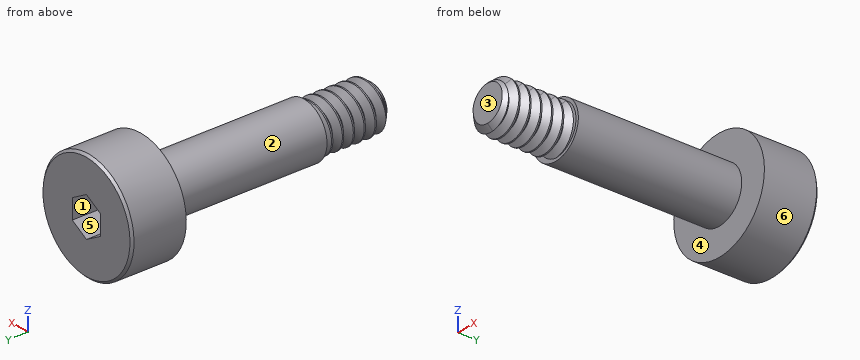
```python
from build123d import *

# Parameters (mm, degrees)
SKETCH1_R          = 3.175
EXTRUDE1_DEPTH     = 3.175
CUT_EXTRUDE1_DEPTH = 1.5875
SKETCH4_R          = 1.5875
EXTRUDE2_DEPTH     = 9.525
SKETCH5_R          = 1.4224
EXTRUDE3_DEPTH     = 3.96875
CHAMFER1_SIZE      = 0.396875
CUT_SWEEP1_PITCH   = 0.635
CUT_SWEEP1_TO      = 3.96875


with BuildPart() as part:
    # Sketch1 → Extrude1 (new body)
    with BuildSketch(Plane(origin=(0, 0, 0), x_dir=(1, 0, 0), z_dir=(0, 1, 0))):
        with Locations(Location((0, 0, 0), (0, 0, 270))):
            Circle(SKETCH1_R)
    extrude(amount=EXTRUDE1_DEPTH)

    # Sketch2 → Cut-Extrude1 (cut)
    with BuildSketch(Plane(origin=(0, 3.175, 0), x_dir=(-1, 0, 0), z_dir=(0, 1, 0))):
        Polygon((0, -1.14567944), (0.9921875, -0.57283972), (0.9921875, 0.57283972), (0, 1.14567944), (-0.9921875, 0.57283972), (-0.9921875, -0.57283972), align=None)
    extrude(amount=-CUT_EXTRUDE1_DEPTH, mode=Mode.SUBTRACT)

    # Sketch4 → Extrude2 (add)
    with BuildSketch(Plane.XZ):
        with Locations(Location((0, 0, 0), (0, 0, 90))):
            Circle(SKETCH4_R)
    extrude(amount=EXTRUDE2_DEPTH)

    # Sketch5 → Extrude3 (add)
    with BuildSketch(Plane.XZ.offset(9.525)):
        with Locations(Location((0, 0, 0), (0, 0, 270))):
            Circle(SKETCH5_R)
    extrude(amount=EXTRUDE3_DEPTH)

    # Chamfer1
    chamfer1_edges = [part.edges().sort_by_distance(p)[0] for p in [
        (0, -13.49375, 1.4224),
    ]]
    chamfer(chamfer1_edges, length=CHAMFER1_SIZE)

    # Cut-Sweep1: arcs per turn and ends read off the stored shape
    # Cut-Sweep1: the profile of Sketch13 profile screwed along a right-hand helix through 7 turns, 6 arcs to a turn; built about Z, then put on its axis
    cut_sweep1_z = Axis((0, 0, 0), (0, 0, 1))
    cut_sweep1_corners = [(1.4227, 0, -0.079201795), (1.4227, 0, -0.635173205), (1.009955401, 0, -0.396875), (1.009955401, 0, -0.3175)]
    with BuildLine(mode=Mode.PRIVATE) as cut_sweep1_profile:
        Line(cut_sweep1_corners[0], cut_sweep1_corners[1])
        Line(cut_sweep1_corners[1], cut_sweep1_corners[2])
        Line(cut_sweep1_corners[2], cut_sweep1_corners[3])
        Line(cut_sweep1_corners[3], cut_sweep1_corners[0])
    cut_sweep1_cap = Face(cut_sweep1_profile.wire())
    cut_sweep1_turn_angles = [0, 30, 60, 90, 120, 150, 180, 210, 240, 270, 300, 330, 360]
    cut_sweep1_turn_weights = [1, 0.8660254037844387, 1, 0.8660254037844387, 1, 0.8660254037844387, 1, 0.8660254037844387, 1, 0.8660254037844387, 1, 0.8660254037844387, 1]
    cut_sweep1_turn_rails = [Edge.make_bspline([Vector(p[0], p[1], 0).rotate(cut_sweep1_z, cut_sweep1_turn_angles[k]) / cut_sweep1_turn_weights[k] + Vector(0, 0, p[2] + CUT_SWEEP1_PITCH * cut_sweep1_turn_angles[k] / 360) for k in range(13)], [0, 0, 0, 1, 1, 2, 2, 3, 3, 4, 4, 5, 5, 6, 6, 6], 2, cut_sweep1_turn_weights) for p in cut_sweep1_corners]
    cut_sweep1_turn_sides = [Face.make_surface_from_curves(cut_sweep1_turn_rails[p[0]], cut_sweep1_turn_rails[p[1]]) for p in [(0, 1), (1, 2), (2, 3), (3, 0)]]
    cut_sweep1 = Plane(origin=(0, -13.49375, 0), x_dir=(0.7071067811865438, 0, 0.7071067811865512), z_dir=(0, 1, 0)) * split(Solid(Shell([*[p.moved(Location((0, 0, CUT_SWEEP1_PITCH * i))) for i in range(7) for p in cut_sweep1_turn_sides], cut_sweep1_cap, cut_sweep1_cap.rotate(cut_sweep1_z, 2520).moved(Location((0, 0, CUT_SWEEP1_PITCH * 2520 / 360)))])), bisect_by=Plane.XY.offset(CUT_SWEEP1_TO), keep=Keep.BOTTOM, mode=Mode.PRIVATE)
    add(cut_sweep1, mode=Mode.SUBTRACT)

    # Sketch11 → Cut-Revolve7 (revolve, cut)
    with BuildSketch(Plane.XY, mode=Mode.PRIVATE) as cut_revolve7_sk:
        Polygon((3.175, 3.045510577), (3.045510577, 3.175), (3.175, 3.175), align=None)
    revolve(cut_revolve7_sk.sketch.rotate(Axis((0, 14.544175091, 0), (0, -1, 0)), 90), axis=Axis((0, 14.544175091, 0), (0, -1, 0)), mode=Mode.SUBTRACT)


solid = part.part
```
Geometry check sheet. Reference: the model listing, model coordinates, mm. Face numbers are marked on the shaded views. A direction names the side the tool comes from. Coordinates: 2 decimals unless noted, no trailing zeros. Write each loop counter-clockwise with the first axis right and the second up, starting at its lowest first coordinate (ties: lowest second). Pieces come first, ordered by that corner, then holes. Notation, with made-up numbers: M 81.25,10.5 L 123.25,10.5 A23 ccw 123.25,37.5 Z; hole C 41,77 d10. An arc over 180 degrees is marked long. Use one line per item in the form item = value. Start each with the question number.
1) Thickness scan on probe 1 along Y at (x, z) = (0.75, 1.25) (3 decimals); probe 2 along Y at (x, z) = (2, -1.75) (3 decimals); probe 3 along Z at (x, y) = (-0.25, 2). Record the ranges inside material, lowest first. Write a range as from..to.
2) Release check for a two-part mould opening along X. For the marked faces 1, 2 and 3 record: pulls with the +X half, pulls with the -X half, needs draft (parallel to the pull), parting line crosses it, or undercut.
3) Section check B-B on y = 1. Enter the section's corners in (x, z) (3 decimals).
4) Set-up check for the marked faces 4, 5 and 6: record each of +Z, -Z, +X, -X, +Y, -Y from which the full face is reachable in a straight line by a thin tool's end or side.
5) Go/stop test with a flat-tipped pin: pin 1 Ø3 at (x, y) = (0, -7) entering from -Z. Record where the tip stops, or that it passes through.
6) Section check A-A on y = -7.25. Enter the section's corners in (x, z) (1 decimal), and give its area (3 significant figures).
Responses:
q1.probe_1 = -9.525..3.175
q1.probe_2 = 0..3.175
q1.probe_3 = -3.17..-1, 1..3.17
q2.face_1 = undercut
q2.face_2 = parting line crosses it
q2.face_3 = needs draft
q3.outline = C 0,0 d6.35
q4.face_4 = -Y
q4.face_5 = +Y
q4.face_6 = +Y, -Y
q5.pin_1 = -1.59
q6.outline = C 0,0 d3.2
q6.area = 7.92 mm2
